Autodesk Inventor part; units mm, degrees
ref_plane "YZ Plane" through (0, 0, 0) normal (1, 0, 0) x (0, 1, 0)
ref_plane "XZ Plane" through (0, 0, 0) normal (0, 1, 0) x (-1, 0, 0)
ref_plane "XY Plane" through (0, 0, 0) normal (0, 0, 1) x (1, 0, 0)
sketch "Sketch1" plane through (0, 0, 0) normal (0, 0, 1) x (1, 0, 0)
  line L0 (0, 0) -> (42.0878, 0)
  line L1 (42.0878, 0) -> (42.0878, 42.0878)
  line L2 (42.0878, 42.0878) -> (0, 42.0878)
  line L3 (0, 42.0878) -> (0, 0)
  dimension "d0" = 42.0878
  dimension "d1" = 42.0878
extrude "Extrusion1" add sketch "Sketch1" along normal blind 1.5748
sketch "Sketch2" plane through (0, 0, 1.5748) normal (0, 0, 1) x (1, 0, 0)
  line L0 (0, 0) -> (42.0878, 0)
  line L1 (42.0878, 0) -> (42.0878, 42.0878)
  line L2 (42.0878, 42.0878) -> (0, 42.0878)
  line L3 (0, 42.0878) -> (0, 0)
  circle A0 centre (5.5104, 36.5774) radius 1.5
  circle A1 centre (36.5774, 36.5774) radius 1.5
  circle A2 centre (36.5774, 5.5104) radius 1.5
  circle A3 centre (5.5104, 5.5104) radius 1.5
  circle A4 centre (12.0142, 26.5938) radius 1.2954
  circle A5 centre (30.0736, 26.5938) radius 1.2954
  circle A6 centre (12.0142, 15.494) radius 1.2954
  circle A7 centre (30.0736, 15.494) radius 1.2954
  dimension "d4" = 3
  dimension "d5" = 2.5908
  dimension "d6" = 28.067
  dimension "d7" = 4.0104
  dimension "d8" = 4.0104
  dimension "d9" = 28.067
  dimension "d10" = 4.0104
  dimension "d11" = 15.4686
  dimension "d12" = 8.509
  dimension "d13" = 10.7188
  dimension "d14" = 10.7188
  dimension "d15" = 14.1986
  dimension "d16" = 14.1986
extrude "Extrusion2" cut sketch "Sketch2" against normal through all contours A0 | A1 | A2 | A3 | A4 | A5 | A6 | A7
sketch "Sketch3" plane through (0, 0, 1.5748) normal (0, 0, 1) x (1, 0, 0)
  line L0 (0, 0) -> (42.0878, 0)
  line L1 (42.0878, 0) -> (42.0878, 42.0878)
  line L2 (42.0878, 42.0878) -> (0, 42.0878)
  line L3 (0, 42.0878) -> (0, 0)
  line L4 (17.8943, 23.622) -> (24.1935, 23.622)
  line L5 (24.1935, 23.622) -> (24.1935, 18.4658)
  line L6 (24.1935, 18.4658) -> (17.8943, 18.4658)
  line L7 (17.8943, 18.4658) -> (17.8943, 23.622)
  dimension "d19" = 6.2992
  dimension "d20" = 5.1562
  dimension "d21" = 18.4658
  dimension "d22" = 18.4658
  dimension "d23" = 17.8943
  dimension "d24" = 17.8943
extrude "Extrusion3" add sketch "Sketch3" along normal blind 1.8796 contours L4 L5 L6 L7
sketch "Sketch4" plane through (0, 0, 3.4544) normal (0, 0, 1) x (1, 0, 0)
  line L0 (24.1935, 23.622) -> (17.8943, 23.622)
  line L1 (17.8943, 23.622) -> (17.8943, 18.4658)
  line L2 (17.8943, 18.4658) -> (24.1935, 18.4658)
  line L3 (24.1935, 18.4658) -> (24.1935, 23.622)
  circle A0 centre (21.0439, 21.0439) radius 2.5781
  point P0 (0, 0)
  dimension "d27" = 3.1496
  dimension "d28" = 3.1496
extrude "Extrusion4" add sketch "Sketch4" along normal blind 0.0254 contours A0
equation "\"d1\" = d0"
equation "\"d7\" = d8"
equation "\"d9\" = d6"
equation "\"d10\" = d8"
equation "\"d13\" = d14"
equation "\"d15\" = d16"
equation "\"d21\" = d22"
equation "\"d23\" = d24"
equation "\"d27\" = d28"
properties part number "Board"
Geometry: final body of the model. Coordinates: model frame, mm. A direction names the side the tool comes from. Coordinates: 2 decimals unless noted, no trailing zeros. Write each loop counter-clockwise with the first axis right and the second up, starting at its lowest first coordinate (ties: lowest second). Pieces come first, ordered by that corner, then holes. Notation, with made-up numbers: (-23, -34) - (30, -34) arc R23 cw to (30, -16) - close; hole circle Ø11 at (39.5, 19.25). An arc over 180 degrees is marked (long way). Return JSON: item names as keys, results as strings.
Item 1: Section query C-C (y = 8). Output: boundary loops of the cut face in (x, z).
Completed:
{"outline": "(0, 0) - (42.09, 0) - (42.09, 1.57) - (0, 1.57) - close"}
Item 2: Section query B-B (z = 1). Count the separate pieces of the cut face and the enclosed holes in it, and give its area (3 significant figures).
Completed:
{"separate pieces": "1", "enclosed holes": "8", "area": "1,720 mm2"}
Item 3: Pin query (flat end, axial travel): pin 1 Ø4 at (x, y) = (5.51, 5.51) entering from +Z; pin 2 Ø0.6 at (y, z) = (20, 2) entering from -X; pin 3 Ø0.6 at (x, z) = (21.5, 2) entering from +Y. Return the tip coordinate at first contact, or that it passes through.
Completed:
{"pin 1": "stops at z = 1.57", "pin 2": "stops at x = 17.89", "pin 3": "stops at y = 23.62"}
Item 4: Line query: L1, parallel to Y at x = 5, z = 1.4; L2, parallel to Y at x = 4.5, z = 0.85; L3, parallel to X at y = 37, z = 1.1. Output: solid intervals per line, ascending.
Completed:
{"L1": "y = 0 to 4.1, 6.92 to 35.17, 37.99 to 42.09", "L2": "y = 0 to 4.4, 6.62 to 35.47, 37.69 to 42.09", "L3": "x = 0 to 4.07, 6.95 to 35.14, 38.02 to 42.09"}
Item 5: Section query A-A (x = 37). Output: boundary loops of the cut face in (y, z), and give its area (3 significant figures).
Completed:
{"outline": "(0, 0) - (4.07, 0) - (4.07, 1.57) - (0, 1.57) - close; (6.95, 0) - (35.14, 0) - (35.14, 1.57) - (6.95, 1.57) - close; (38.02, 0) - (42.09, 0) - (42.09, 1.57) - (38.02, 1.57) - close", "area": "57.2 mm2"}
Item 6: Reachability of faces 1 (the face through (24.194, 21, 3)), 2 (the face through (31.31, 26.98, 0.8)), 3 (the face through (21, 18.466, 3)), 4 (the face through (17.894, 21, 3)) from +Z, -Z, +X, -X, +Y, -Y: full face, straight path, thin tool, end or side. Return the list, or none.
Completed:
{"face 1": "+Z, +X, +Y, -Y", "face 2": "+Z, -Z", "face 3": "+Z, +X, -X, -Y", "face 4": "+Z, -X, +Y, -Y"}
